Verification items for the finished model (mm, model axes). A direction names the side the tool comes from. Round coordinates to 2 decimals unless told otherwise and drop trailing zeros. Order: outer loops, then holes, each group sorted by start corner. A loop starts at its lowest first (then second) coordinate and runs counter-clockwise, first axis right, second up.
```python
from build123d import *

# Parameters (mm, degrees)
F3_R     = 2.9977693339
F4_DEPTH = 2.5
F5_R     = 5.1348432566
F6_DEPTH = 2.5


with BuildPart() as f2:
    # F2: sweep along a path in F1
    with BuildLine(Plane.YZ) as f2_path:
        Line((0, -35.2961234748), (90, -35.2961234748))
        ThreePointArc((90, -35.2961234748), (97.0710678119, -38.225055663), (100, -45.2961234748))
        Line((100, -45.2961234748), (100, -85.2961234748))
        ThreePointArc((100, -85.2961234748), (97.0710678119, -92.3671912867), (90, -95.2961234748))
        Line((90, -95.2961234748), (0, -95.2961234748))
    # F0 (on Front) → F2 (sweep)
    with BuildSketch(Plane.XZ):
        with BuildLine():
            Line((16.2149220705, 35.2961234748), (0, 35.2961234748))
            Line((0, 35.2961234748), (-16.2149220705, 35.2961234748))
            Line((-16.2149220705, 35.2961234748), (-16.2149220705, 30.2961234748))
            Line((-16.2149220705, 30.2961234748), (-5.5, 30.2961234748))
            ThreePointArc((-5.5, 30.2961234748), (-3.3786796564, 29.4174438184), (-2.5, 27.2961234748))
            Line((-2.5, 27.2961234748), (-2.5, 0))
            Line((-2.5, 0), (-2.5, -27.2961234748))
            ThreePointArc((-2.5, -27.2961234748), (-3.3786796564, -29.4174438184), (-5.5, -30.2961234748))
            Line((-5.5, -30.2961234748), (-16.2149220705, -30.2961234748))
            Line((-16.2149220705, -30.2961234748), (-16.2149220705, -35.2961234748))
            Line((-16.2149220705, -35.2961234748), (0, -35.2961234748))
            Line((0, -35.2961234748), (16.2149220705, -35.2961234748))
            Line((16.2149220705, -35.2961234748), (16.2149220705, -30.2961234748))
            Line((16.2149220705, -30.2961234748), (5.5, -30.2961234748))
            ThreePointArc((5.5, -30.2961234748), (3.3786796564, -29.4174438184), (2.5, -27.2961234748))
            Line((2.5, -27.2961234748), (2.5, 0))
            Line((2.5, 0), (2.5, 27.2961234748))
            ThreePointArc((2.5, 27.2961234748), (3.3786796564, 29.4174438184), (5.5, 30.2961234748))
            Line((5.5, 30.2961234748), (16.2149220705, 30.2961234748))
            Line((16.2149220705, 30.2961234748), (16.2149220705, 35.2961234748))
        make_face()
    sweep(path=f2_path.line)

    # F3 (on Right) → F4 (join, symmetric)
    with BuildSketch(Plane.YZ):
        with BuildLine():
            Line((0, 65.2961234748), (0, 35.2961234748))
            Line((0, 35.2961234748), (70, 35.2961234748))
            Line((70, 35.2961234748), (15.5028312053, 72.1644029996))
            ThreePointArc((15.5028312053, 72.1644029996), (5.8488593767, 73.0246440824), (0, 65.2961234748))
        make_face()
        with Locations((9.8994718868, 63.8817485732)):
            Circle(F3_R, mode=Mode.SUBTRACT)
    extrude(amount=F4_DEPTH, both=True)

    # F5 (on Right) → F6 (join, symmetric)
    with BuildSketch(Plane.YZ):
        with BuildLine():
            Line((70, -165.8883704245), (0, -165.8883704245))
            Line((0, -165.8883704245), (0, -195.8883704245))
            ThreePointArc((0, -195.8883704245), (6.1459122057, -202.2103795466), (14.9061395374, -201.2111532078))
            Line((14.9061395374, -201.2111532078), (70, -165.8883704245))
        make_face()
        with Locations((9.508806352, -192.7927926497)):
            Circle(F5_R, mode=Mode.SUBTRACT)
    extrude(amount=F6_DEPTH, both=True)


solid = f2.part
```
1) Sectioned sample at B-B on z = -79. Record the cut outline in (x, y).
2) Scan lines: probe 1 along Z at (x, y) = (10.5, 81.5); probe 2 along Y at (x, z) = (9.5, -82.5); probe 3 along Z at (x, y) = (-4.5, 80). Record each from-to range of solid material in increasing order.
3) Sectioned sample at A-A on x = -9.5. Record the cut outline in (y, z).
4) Tool access check on faces 4 (the flat face through (-11, 46, -30.296)), 5 (the flat face through (11, 46, -30.296)), 6 (the flat face through (2.5, 119, -67)). Record the directions out of +Z, -Z, +X, -X, +Y, -Y that give a thin tool (end or side, any length) a straight path to the whole face; none if there is none.
5) Go/stop test with flat-tipped pins: pin 1 Ø1 at (x, z) = (-9, -116) entering from +Y; pin 2 Ø12 at (x, y) = (-11, 38) entering from -Z; pin 3 Ø10 at (x, y) = (3.5, 116.5) entering from +Z; pin 4 Ø12 at (y, z) = (39.5, -158) entering from -X. Record where each tip stops, or that it passes through.
6) Draft check along Y on faces 1 (the cylindrical face through (0.227, 96.993, -38.148)), 2 (the flat face through (11, 105, -66)), 3 (the flat face through (2.5, 27, 51)). Enter one of: released by +Y, released by -Y, zero draft, split by the parting line, or undercut.
Returned:
1. outline: (-16.21, 100) - (16.21, 100) - (16.21, 105) - (5.5, 105) arc R3 cw to (2.5, 108) - (2.5, 162.59) arc R3 cw to (5.5, 165.59) - (16.21, 165.59) - (16.21, 170.59) - (-16.21, 170.59) - (-16.21, 165.59) - (-5.5, 165.59) arc R3 cw to (-2.5, 162.59) - (-2.5, 108) arc R3 cw to (-5.5, 105) - (-16.21, 105) - close
2. probe 1: z = -165.89 to -160.89, -100.3 to -95.3, -35.3 to -30.3, 30.3 to 35.3
2. probe 2: y = 100 to 105, 165.59 to 170.59
2. probe 3: z = -165.89 to -160.72, -100.47 to -95.3, -35.3 to -30.12, 30.12 to 35.3
3. outline: (0, -165.89) - (90, -165.89) arc R80.59 ccw to (170.59, -85.3) - (170.59, -45.3) arc R80.59 ccw to (90, 35.3) - (0, 35.3) - (0, 30.3) - (90, 30.3) arc R75.59 cw to (165.59, -45.3) - (165.59, -85.3) arc R75.59 cw to (90, -160.89) - (0, -160.89) - close; (0, -100.3) - (90, -100.3) arc R15 ccw to (105, -85.3) - (105, -45.3) arc R15 ccw to (90, -30.3) - (0, -30.3) - (0, -35.3) - (90, -35.3) arc R10 cw to (100, -45.3) - (100, -85.3) arc R10 cw to (90, -95.3) - (0, -95.3) - close
4. face 4: -X, -Y
4. face 5: +X, -Y
4. face 6: +X
5. pin 1: stops at y = 164.72
5. pin 2: stops at z = -165.89
5. pin 3: stops at z = 32.38
5. pin 4: stops at x = -16.21
6. face 1: released by -Y
6. face 2: undercut
6. face 3: zero draft
